Geometry: see drawing. Coordinates: mm, zero at the bounding-box minimum. A direction names the side the tool comes from. Give positions to 0.01 mm unless a question says otherwise; leave off trailing zeros. Write each loop counter-clockwise with the first axis right and the second up, starting at its lowest first coordinate (ties: lowest second). Pieces come first, ordered by that corner, then holes. Notation, with made-up numbers: M -5.75,26 L 41.25,26 A6 ccw 41.25,37 Z; hole C 41.25,-38 d8. An arc over 180 degrees is marked long. Use one line per item in the form item = value. Start each with the question number.
Item 1: Section query C-C on x = 2.25. Return loops of the section in (y, z).
Item 2: Section query A-A on z = 2. Return loops of the section in (x, y), then the cut area to 3 significant figures.
Item 3: Contact query for flat-ended pins moving along their axis: P1, Ø2.5, axis at x = 2.25, y = 4.5, coming from the +Z side; P2, Ø1.3, axis at x = 1.5, y = 5.5, coming from the -Z side. Output: stop coordinate, or through.
Item 4: Section query D-D on x = 4.1. Return loops of the section in (y, z), then the cut area to 3 significant figures.
Item 5: Material intervals for line 1 along X through (y, z) = (1.25, 2); line 2 along Y through (x, z) = (2.25, 7.15); line 3 along Y through (x, z) = (4.3, 1), sorted ascending. Write a range as from..to.
Item 6: Section query B-B on y = 4.5. Return loops of the section in (x, z), then the cut area to 3 significant figures.
Item 7: Access query for the marked faces 1 and 2. Directions: +Z, -Z, +X, -X, +Y, -Y. A direction counts if a zero-diameter tool reaches every point of the face in a straight line with its end or side. Return the directions, or none.
Item 8: Pull-direction query (Y, two-part tool) for the marked faces 3, 4 and 5; classes: released by +Y, released by -Y, zero draft, split by the parting line, or undercut.
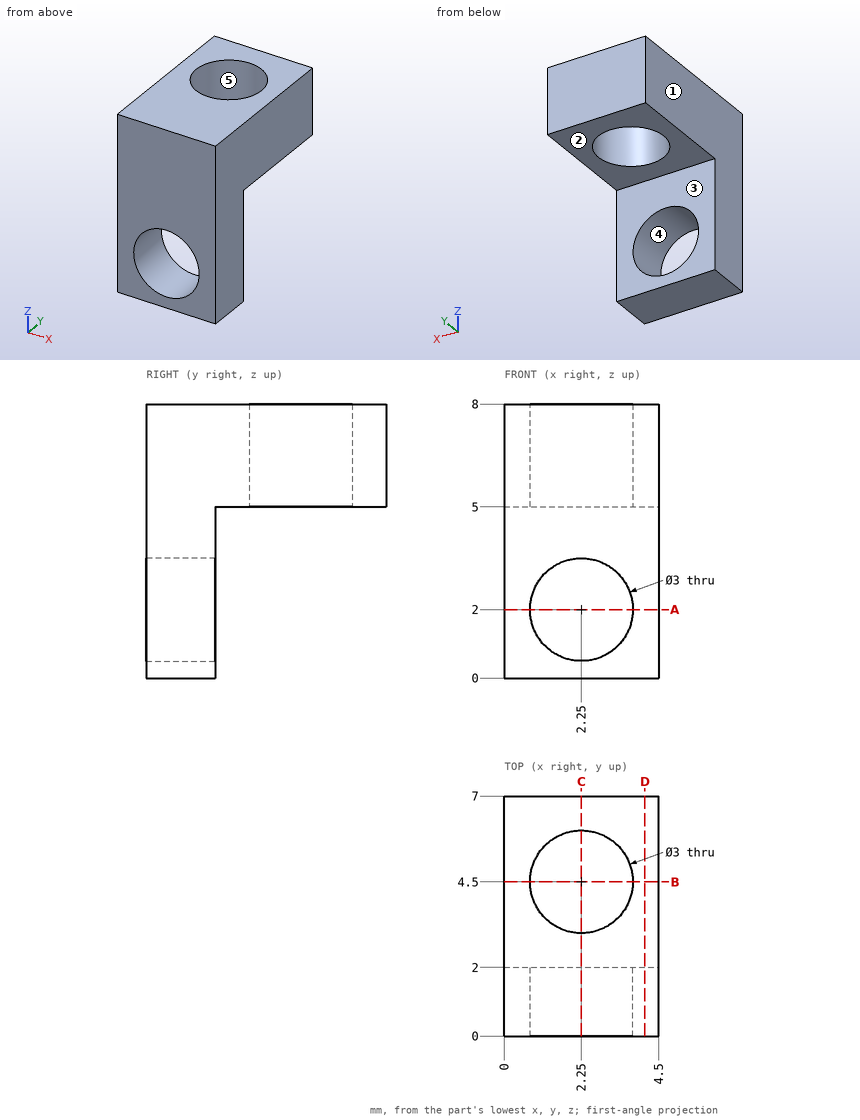
Answer sheet:
q1.outline = M 0,0 L 2,0 L 2,0.5 L 0,0.5 Z; M 0,3.5 L 2,3.5 L 2,5 L 3,5 L 3,8 L 0,8 Z; M 6,5 L 7,5 L 7,8 L 6,8 Z
q2.outline = M 0,0 L 0.75,0 L 0.75,2 L 0,2 Z; M 3.75,0 L 4.5,0 L 4.5,2 L 3.75,2 Z
q2.area = 3.00 mm2
q3.P1 = through
q3.P2 = 5
q4.outline = M 0,0 L 2,0 L 2,5 L 7,5 L 7,8 L 0,8 Z
q4.area = 31.0 mm2
q5.line_1 = 0..0.75, 3.75..4.5
q5.line_2 = 0..3, 6..7
q5.line_3 = 0..2
q6.outline = M 0,5 L 0.75,5 L 0.75,8 L 0,8 Z; M 3.75,5 L 4.5,5 L 4.5,8 L 3.75,8 Z
q6.area = 4.50 mm2
q7.face_1 = +Z, -Z, -X, +Y, -Y
q7.face_2 = -Z, +X, -X, +Y
q8.face_3 = released by +Y
q8.face_4 = zero draft
q8.face_5 = undercut
